```python
from build123d import *

# Parameters (mm, degrees)
SKETCH1_R      = 3.4
EXTRUDE1_DEPTH = 300


with BuildPart() as part:
    # Sketch1 → Extrude1 (new body)
    with BuildSketch(Plane.XY):
        with BuildLine():
            Line((7.685, 3.358241745), (7.685, -3.358241745))
            ThreePointArc((7.685, -3.358241745), (8.046005845, -5.174620093), (9.074149602, -6.714904463))
            Line((9.074149602, -6.714904463), (12.373454754, -10.018325737))
            ThreePointArc((12.373454754, -10.018325737), (12.662327453, -10.211539726), (13.003171987, -10.279393143))
            Line((13.003171987, -10.279393143), (15.298849809, -10.279393143))
            ThreePointArc((15.298849809, -10.279393143), (16.196875422, -9.907418755), (16.568849809, -9.009393143))
            Line((16.568849809, -9.009393143), (16.568849809, -6.901425905))
            Line((16.568849809, -6.901425905), (15.94, -6.901425905))
            Line((15.94, -6.901425905), (15.94, -5.758104362))
            ThreePointArc((15.94, -5.758104362), (16.399842354, -4.647946715), (17.51, -4.188104362))
            Line((17.51, -4.188104362), (18.43, -4.188104362))
            ThreePointArc((18.43, -4.188104362), (19.540157646, -4.647946715), (20, -5.758104362))
            Line((20, -5.758104362), (20, -13.186220555))
            Line((20, -13.186220555), (20, -16.83))
            ThreePointArc((20, -16.83), (19.071528496, -19.071528496), (16.83, -20))
            Line((16.83, -20), (13.004526429, -20))
            Line((13.004526429, -20), (5.63, -20))
            ThreePointArc((5.63, -20), (4.519842354, -19.540157646), (4.06, -18.43))
            Line((4.06, -18.43), (4.06, -17.696220555))
            ThreePointArc((4.06, -17.696220555), (4.519842354, -16.586062909), (5.63, -16.126220555))
            Line((5.63, -16.126220555), (6.7839284, -16.126220555))
            Line((6.7839284, -16.126220555), (6.7839284, -16.886683809))
            Line((6.7839284, -16.886683809), (9.015, -16.886683809))
            ThreePointArc((9.015, -16.886683809), (9.913025612, -16.514709421), (10.285, -15.616683809))
            Line((10.285, -15.616683809), (10.285, -12.922193682))
            ThreePointArc((10.285, -12.922193682), (10.254851172, -12.69250702), (10.166447275, -12.47838167))
            Line((10.166447275, -12.47838167), (6.770639403, -9.078337282))
            ThreePointArc((6.770639403, -9.078337282), (5.228903087, -8.047139023), (3.409789005, -7.685))
            Line((3.409789005, -7.685), (-3.409789005, -7.685))
            ThreePointArc((-3.409789005, -7.685), (-5.228903087, -8.047139023), (-6.770639403, -9.078337282))
            Line((-6.770639403, -9.078337282), (-10.166447275, -12.47838167))
            ThreePointArc((-10.166447275, -12.47838167), (-10.254851172, -12.69250702), (-10.285, -12.922193682))
            Line((-10.285, -12.922193682), (-10.285, -15.616683809))
            ThreePointArc((-10.285, -15.616683809), (-9.913025612, -16.514709421), (-9.015, -16.886683809))
            Line((-9.015, -16.886683809), (-6.7839284, -16.886683809))
            Line((-6.7839284, -16.886683809), (-6.7839284, -16.126220555))
            Line((-6.7839284, -16.126220555), (-5.63, -16.126220555))
            ThreePointArc((-5.63, -16.126220555), (-4.519842354, -16.586062909), (-4.06, -17.696220555))
            Line((-4.06, -17.696220555), (-4.06, -18.43))
            ThreePointArc((-4.06, -18.43), (-4.519842354, -19.540157646), (-5.63, -20))
            Line((-5.63, -20), (-13.004526429, -20))
            Line((-13.004526429, -20), (-16.83, -20))
            ThreePointArc((-16.83, -20), (-19.071528496, -19.071528496), (-20, -16.83))
            Line((-20, -16.83), (-20, -13.186220555))
            Line((-20, -13.186220555), (-20, -5.758104362))
            ThreePointArc((-20, -5.758104362), (-19.540157646, -4.647946715), (-18.43, -4.188104362))
            Line((-18.43, -4.188104362), (-17.51, -4.188104362))
            ThreePointArc((-17.51, -4.188104362), (-16.399842354, -4.647946715), (-15.94, -5.758104362))
            Line((-15.94, -5.758104362), (-15.94, -6.901425905))
            Line((-15.94, -6.901425905), (-16.568849809, -6.901425905))
            Line((-16.568849809, -6.901425905), (-16.568849809, -9.009393143))
            ThreePointArc((-16.568849809, -9.009393143), (-16.196875422, -9.907418755), (-15.298849809, -10.279393143))
            Line((-15.298849809, -10.279393143), (-13.003171987, -10.279393143))
            ThreePointArc((-13.003171987, -10.279393143), (-12.662327453, -10.211539726), (-12.373454754, -10.018325737))
            Line((-12.373454754, -10.018325737), (-9.074149602, -6.714904463))
            ThreePointArc((-9.074149602, -6.714904463), (-8.046005845, -5.174620093), (-7.685, -3.358241745))
            Line((-7.685, -3.358241745), (-7.685, 3.358241745))
            ThreePointArc((-7.685, 3.358241745), (-8.046005845, 5.174620093), (-9.074149602, 6.714904463))
            Line((-9.074149602, 6.714904463), (-12.373454754, 10.018325737))
            ThreePointArc((-12.373454754, 10.018325737), (-12.662327453, 10.211539726), (-13.003171987, 10.279393143))
            Line((-13.003171987, 10.279393143), (-15.298849809, 10.279393143))
            ThreePointArc((-15.298849809, 10.279393143), (-16.196875422, 9.907418755), (-16.568849809, 9.009393143))
            Line((-16.568849809, 9.009393143), (-16.568849809, 6.901425905))
            Line((-16.568849809, 6.901425905), (-15.94, 6.901425905))
            Line((-15.94, 6.901425905), (-15.94, 5.758104362))
            ThreePointArc((-15.94, 5.758104362), (-16.399842354, 4.647946715), (-17.51, 4.188104362))
            Line((-17.51, 4.188104362), (-18.43, 4.188104362))
            ThreePointArc((-18.43, 4.188104362), (-19.540157646, 4.647946715), (-20, 5.758104362))
            Line((-20, 5.758104362), (-20, 13.186220555))
            Line((-20, 13.186220555), (-20, 16.83))
            ThreePointArc((-20, 16.83), (-19.071528496, 19.071528496), (-16.83, 20))
            Line((-16.83, 20), (-13.004526429, 20))
            Line((-13.004526429, 20), (-5.63, 20))
            ThreePointArc((-5.63, 20), (-4.519842354, 19.540157646), (-4.06, 18.43))
            Line((-4.06, 18.43), (-4.06, 17.696220555))
            ThreePointArc((-4.06, 17.696220555), (-4.519842354, 16.586062909), (-5.63, 16.126220555))
            Line((-5.63, 16.126220555), (-6.7839284, 16.126220555))
            Line((-6.7839284, 16.126220555), (-6.7839284, 16.886683809))
            Line((-6.7839284, 16.886683809), (-9.015, 16.886683809))
            ThreePointArc((-9.015, 16.886683809), (-9.913025612, 16.514709421), (-10.285, 15.616683809))
            Line((-10.285, 15.616683809), (-10.285, 12.922193682))
            ThreePointArc((-10.285, 12.922193682), (-10.254851172, 12.69250702), (-10.166447275, 12.47838167))
            Line((-10.166447275, 12.47838167), (-6.770639403, 9.078337282))
            ThreePointArc((-6.770639403, 9.078337282), (-5.228903087, 8.047139023), (-3.409789005, 7.685))
            Line((-3.409789005, 7.685), (3.409789005, 7.685))
            ThreePointArc((3.409789005, 7.685), (5.228903087, 8.047139023), (6.770639403, 9.078337282))
            Line((6.770639403, 9.078337282), (10.166447275, 12.47838167))
            ThreePointArc((10.166447275, 12.47838167), (10.254851172, 12.69250702), (10.285, 12.922193682))
            Line((10.285, 12.922193682), (10.285, 15.616683809))
            ThreePointArc((10.285, 15.616683809), (9.913025612, 16.514709421), (9.015, 16.886683809))
            Line((9.015, 16.886683809), (6.7839284, 16.886683809))
            Line((6.7839284, 16.886683809), (6.7839284, 16.126220555))
            Line((6.7839284, 16.126220555), (5.63, 16.126220555))
            ThreePointArc((5.63, 16.126220555), (4.519842354, 16.586062909), (4.06, 17.696220555))
            Line((4.06, 17.696220555), (4.06, 18.43))
            ThreePointArc((4.06, 18.43), (4.519842354, 19.540157646), (5.63, 20))
            Line((5.63, 20), (13.004526429, 20))
            Line((13.004526429, 20), (16.83, 20))
            ThreePointArc((16.83, 20), (19.071528496, 19.071528496), (20, 16.83))
            Line((20, 16.83), (20, 13.186220555))
            Line((20, 13.186220555), (20, 5.758104362))
            ThreePointArc((20, 5.758104362), (19.540157646, 4.647946715), (18.43, 4.188104362))
            Line((18.43, 4.188104362), (17.51, 4.188104362))
            ThreePointArc((17.51, 4.188104362), (16.399842354, 4.647946715), (15.94, 5.758104362))
            Line((15.94, 5.758104362), (15.94, 6.901425905))
            Line((15.94, 6.901425905), (16.568849809, 6.901425905))
            Line((16.568849809, 6.901425905), (16.568849809, 9.009393143))
            ThreePointArc((16.568849809, 9.009393143), (16.196875422, 9.907418755), (15.298849809, 10.279393143))
            Line((15.298849809, 10.279393143), (13.003171987, 10.279393143))
            ThreePointArc((13.003171987, 10.279393143), (12.662327453, 10.211539726), (12.373454754, 10.018325737))
            Line((12.373454754, 10.018325737), (9.074149602, 6.714904463))
            ThreePointArc((9.074149602, 6.714904463), (8.046005845, 5.174620093), (7.685, 3.358241745))
        make_face()
        Circle(SKETCH1_R, mode=Mode.SUBTRACT)
        with BuildLine():
            Line((12.57, 18.35), (15.55, 18.35))
            ThreePointArc((15.55, 18.35), (17.529898987, 17.529898987), (18.35, 15.55))
            Line((18.35, 15.55), (18.35, 12.57))
            ThreePointArc((18.35, 12.57), (18.165477272, 12.124522728), (17.72, 11.94))
            Line((17.72, 11.94), (13.21, 11.94))
            ThreePointArc((13.21, 11.94), (12.311974388, 12.311974388), (11.94, 13.21))
            Line((11.94, 13.21), (11.94, 17.72))
            ThreePointArc((11.94, 17.72), (12.124522728, 18.165477272), (12.57, 18.35))
        make_face(mode=Mode.SUBTRACT)
        with BuildLine():
            Line((-12.57, -18.35), (-15.55, -18.35))
            ThreePointArc((-15.55, -18.35), (-17.529898987, -17.529898987), (-18.35, -15.55))
            Line((-18.35, -15.55), (-18.35, -12.57))
            ThreePointArc((-18.35, -12.57), (-18.165477272, -12.124522728), (-17.72, -11.94))
            Line((-17.72, -11.94), (-13.21, -11.94))
            ThreePointArc((-13.21, -11.94), (-12.311974388, -12.311974388), (-11.94, -13.21))
            Line((-11.94, -13.21), (-11.94, -17.72))
            ThreePointArc((-11.94, -17.72), (-12.124522728, -18.165477272), (-12.57, -18.35))
        make_face(mode=Mode.SUBTRACT)
        with BuildLine():
            Line((18.35, -15.55), (18.35, -12.57))
            ThreePointArc((18.35, -12.57), (18.165477272, -12.124522728), (17.72, -11.94))
            Line((17.72, -11.94), (13.21, -11.94))
            ThreePointArc((13.21, -11.94), (12.311974388, -12.311974388), (11.94, -13.21))
            Line((11.94, -13.21), (11.94, -17.72))
            ThreePointArc((11.94, -17.72), (12.124522728, -18.165477272), (12.57, -18.35))
            Line((12.57, -18.35), (15.55, -18.35))
            ThreePointArc((15.55, -18.35), (17.529898987, -17.529898987), (18.35, -15.55))
        make_face(mode=Mode.SUBTRACT)
        with BuildLine():
            Line((-18.35, 15.55), (-18.35, 12.57))
            ThreePointArc((-18.35, 12.57), (-18.165477272, 12.124522728), (-17.72, 11.94))
            Line((-17.72, 11.94), (-13.21, 11.94))
            ThreePointArc((-13.21, 11.94), (-12.311974388, 12.311974388), (-11.94, 13.21))
            Line((-11.94, 13.21), (-11.94, 17.72))
            ThreePointArc((-11.94, 17.72), (-12.124522728, 18.165477272), (-12.57, 18.35))
            Line((-12.57, 18.35), (-15.55, 18.35))
            ThreePointArc((-15.55, 18.35), (-17.529898987, 17.529898987), (-18.35, 15.55))
        make_face(mode=Mode.SUBTRACT)
    extrude(amount=-EXTRUDE1_DEPTH)


solid = part.part
```
The listing builds one solid part. Answer for the finished solid, in the listing's coordinates (mm). A direction names the side the tool comes from. Give positions to 0.01 mm unless a question says otherwise; leave off trailing zeros. Order: outer loops, then holes, each group sorted by start corner. A loop starts at its lowest first (then second) coordinate and runs counter-clockwise, first axis right, second up. Notation, with made-up numbers: (57.5, 11) -> (64.5, 11) arc R24 ccw to (64.5, 26) -> close; hole circle Ø9 at (19, -7). An arc over 180 degrees is marked (long way). One line per item, written item: value.
1) Flat-ended cylindrical pins translate along their axes: P1, Ø7.5, axis at y = 0, z = -194.5, coming from the -X side; P2, Ø5, axis at x = 12.5, y = -2, coming from the +Z side; P3, Ø4, axis at x = -3, z = -75.5, coming from the -Y side; P4, Ø0.6, axis at y = -18, z = -95.5, coming from the -X side. Find the tip coordinate at first contact, or state that the pin passes through.
Reported:
P1: stops at x = -7.7
P2: passes through
P3: stops at y = -19.87
P4: stops at x = -19.88
2) Find the intervals of material crossed by line 1 (X direction, y = -8.5, z = -143); line 2 (Y direction, x = -12.5, z = -207.5); line 3 (Y direction, x = 0, z = -118) (3 decimals), in increasing order.
Reported:
line 1: x = -20 to -16.57, -10.86 to -6.07, 6.07 to 10.86, 16.57 to 20
line 2: y = -20 to -18.35, -12.16 to -10.12, 10.12 to 12.16, 18.35 to 20
line 3: y = -7.685 to -3.4, 3.4 to 7.685
3) Determine the mould class of faces 4 (the flat face through (11, -20, -148)), 5 (the flat face through (20, 11, -148)), 6 (the flat face through (0, 7.685, -148)), 7 (the flat face through (7.685, 0, -148)) for opening direction Y: pulls with the +Y half, pulls with the -Y half, needs draft (parallel to the pull), parting line crosses it, or undercut.
Reported:
face 4: pulls with the -Y half
face 5: needs draft
face 6: pulls with the +Y half
face 7: undercut
4) Find section A-A, the plane y = 0. Determine the outline of the cut face in (x, z) (3 decimals).
Reported:
outline: (-7.685, -300) -> (-3.4, -300) -> (-3.4, 0) -> (-7.685, 0) -> close; (3.4, -300) -> (7.685, -300) -> (7.685, 0) -> (3.4, 0) -> close
5) A tool of negligible diameter and unlimited length cuts with its end or side. For faces 1 (the flat face through (0, -7.685, -148)), 2 (the flat face through (2, 3, -300)), 3 (the flat face through (-7.685, 0, -148)), from which of +Z, -Z, +X, -X, +Y, -Y can it reach the whole face along a straight path? Write none if from no direction.
Reported:
face 1: +Z, -Z, -Y
face 2: -Z, +X, -X, +Y, -Y
face 3: +Z, -Z, -X
6) Find section C-C, the plane z = -122. Count the separate pieces of the cut face and the enclosed holes in it, plus the area to 3 significant figures.
Reported:
separate pieces: 1
enclosed holes: 5
area: 658 mm^2
